from build123d import *

# Parameters (mm, degrees)
F2_T = -1.2


with BuildPart() as f1:
    # F0 (on Front) → F1 (revolve)
    with BuildSketch(Plane.XZ):
        Polygon((0, 9.676), (0, 0), (4.318, 0), (4.318, 3.81), (7.366, 3.81), (7.366, 4.31), (2, 9.676), align=None)
    revolve(axis=Axis((0, 0, 4.838), (0, 0, -1)))

    # F2
    f2_openings = [f1.faces().sort_by_distance(p)[0] for p in [
        (0, 0, 0),
    ]]
    offset(amount=F2_T, openings=f2_openings, kind=Kind.INTERSECTION)

    # F3 (on Front) → F4 (revolve)
    with BuildSketch(Plane.XZ):
        Polygon((4.9689437252, 5.01), (3.118, 6.8609437252), (3.118, 5.01), align=None)
    revolve(axis=Axis((0, 0, 0), (0, 0, 1)))


solid = f1.part
The listing builds one solid part. Answer for the finished solid, in the listing's coordinates (mm). A direction names the side the tool comes from. Round coordinates to 2 decimals unless told otherwise and drop trailing zeros. Loops run counter-clockwise (first coordinate to the right, second up) from the corner with the lowest first, then second, coordinate; pieces in that order, holes last. Notation, with made-up numbers: M 18,50 L 31,50 A16 ccw 31,54 Z; hole C 67.5,-28 d1. An arc over 180 degrees is marked long. Write each question's results on one line, items separated by ' | '. Start each with the question number.
1) Determine the mould class of faces 3 (the flat face through (-3, 2, 0)), 4 (the cylindrical face through (1.676, 2.629, 3.382)), 5 (the cylindrical face through (3.399, 6.535, 4.063)) for opening direction X: pulls with the +X half, pulls with the -X half, needs draft (parallel to the pull), parting line crosses it, or undercut.
2) Which of the six approach directions +Z, -Z, +X, -X, +Y, -Y give full straight-line access (tool end or side, diameter ignored) to faces 1 (the conical face through (-1.794, 1.376, 9.415)), 2 (the flat face through (0, 0, 8.476))?
3) Find section A-A on y = 0. Write down the section's boundary in (x, z), plus the area to 3 significant figures.
4) Find section C-C on z = 1.25. Write down the section's boundary in (x, y).
5) Straight lines are drawn through the part: probe 1 along Y at (x, z) = (0, 4); probe 2 along Y at (x, z) = (0, 3.5); probe 3 along Z at (x, y) = (-1.25, -1.5). For each, find the intervals that lie inside material, in ascending order.
6) Each of these flat-tipped pins is pushed along its axis until it touches: pin 1 (5 mm diameter, centred on x = 4.5, y = 2, fed in from +Z); pin 2 (7 mm diameter, centred on x = 0, y = 0, fed in from -Z); pin 3 (3 mm diameter, centred on x = -0.5, y = 4.5, fed in from +Z); pin 4 (2 mm diameter, centred on x = -0.5, y = -3.5, fed in from +Z). Where does it stop, or does it pass through?
7) Find section D-D on z = 4.75. Write down the section's boundary in (x, y), plus the area to 3 significant figures.
Final values:
1) face 3: needs draft | face 4: undercut | face 5: parting line crosses it
2) face 1: +Z | face 2: -Z
3) outline: M -7.37,3.81 L -4.32,3.81 L -4.32,0 L -3.12,0 L -3.12,6.86 L -1.5,8.48 L 1.5,8.48 L 3.12,6.86 L 3.12,0 L 4.32,0 L 4.32,3.81 L 7.37,3.81 L 7.37,4.31 L 2,9.68 L -2,9.68 L -7.37,4.31 Z | area: 40.3 mm²
4) outline: C 0,0 d8.64; hole C 0,0 d6.24
5) probe 1: -7.37 to -3.12, 3.12 to 7.37 | probe 2: -4.32 to -3.12, 3.12 to 4.32 | probe 3: 8.03 to 9.68
6) pin 1: z = 9.25 | pin 2: z = 0 | pin 3: z = 8.65 | pin 4: z = 9.14
7) outline: C 0,0 d13.85; hole C 0,0 d6.24 | area: 120 mm²
